Autodesk Inventor part; units mm, degrees
ref_plane "Work Plane2" through (-142.9124, -40, 12) normal (0, 0, 1) x (1, 0, 0)
ref_plane "YZ Plane" through (0, 0, 0) normal (1, 0, 0) x (0, 1, 0)
ref_plane "XZ Plane" through (0, 0, 0) normal (0, 1, 0) x (-1, 0, 0)
ref_plane "Work Plane1" through (0, 0, 0) normal (0, 0, 1) x (1, 0, 0)
sketch "Sketch1" plane through (0, 0, 0) normal (0, 0, 1) x (1, 0, 0)
  circle A0 centre (13.9438, -25.4) radius 3.3782 construction
  line L0 (31.1796, -40) -> (-0.106, -40) construction
  line L1 (31.1796, -40) -> (31.1796, -8.95) construction
  line L2 (31.1796, -8.95) -> (23.5548, -8.95) construction
  line L3 (23.5548, -8.95) -> (23.5548, -10.525) construction
  line L4 (23.5548, -10.525) -> (12.648, -10.525) construction
  line L5 (12.648, -10.525) -> (12.648, -8.95) construction
  line L6 (12.648, -8.95) -> (-0.106, -8.95) construction
  line L7 (-0.106, -8.95) -> (-0.106, -40) construction
  circle A1 centre (13.9438, 25.4) radius 3.3782 construction
  line L8 (-0.106, 8.95) -> (12.648, 8.95) construction
  line L9 (12.648, 8.95) -> (12.648, 10.525) construction
  line L10 (12.648, 10.525) -> (23.5548, 10.525) construction
  line L11 (23.5548, 10.525) -> (23.5548, 8.95) construction
  line L12 (23.5548, 8.95) -> (31.1796, 8.95) construction
  line L13 (31.1796, 8.95) -> (31.1796, 45) construction
  line L14 (-0.106, 45) -> (31.1796, 45) construction
  line L15 (-0.106, 45) -> (-0.106, 8.95) construction
  line L16 (31.1796, -18.5) -> (-0.106, -18.5)
  line L17 (-0.106, -18.5) -> (-0.106, 18.5)
  line L18 (-0.106, 18.5) -> (31.1796, 18.5)
  line L19 (31.1796, 18.5) -> (31.1796, -18.5)
  line L20 (65.998, 0) -> (-177.7308, 0) construction
  circle A2 centre (13.9438, 25.4) radius 5.5 construction
  circle A3 centre (23.1796, -13.5) radius 2
  circle A4 centre (7.894, -13.5) radius 2
  circle A5 centre (7.894, 13.5) radius 2
  circle A6 centre (23.1796, 13.5) radius 2
  point P0 (0, 0)
  point P1 (13.9438, 22.0218)
  dimension "d2" = 37
  dimension "d3" = 11
ref_plane "Work Plane2" through (-142.9124, -40, 12) normal (0, 0, 1) x (1, 0, 0)
extrude "Extrusion1" add sketch "Sketch1" along normal up to surface (12 mm away) contours L16 L17 L18 L19 | A3 | A4 | A5 | A6
sketch "Sketch2" plane through (0, 0, 0) normal (0, 1, 0) x (-1, 0, 0)
  line L0 (1.106, -8.95) -> (1.106, 0)
  line L1 (1.106, 0) -> (-32.1796, 0)
  line L2 (-32.1796, 0) -> (-32.1796, -8.95)
  line L3 (-38.8367, 0) -> (7.7631, 0) construction
  line L4 (-31.1796, -8.95) -> (-31.1796, 0) construction
  line L5 (0.106, 7.5245) -> (0.106, -7.5245) construction
  line L6 (-31.1796, -8.95) -> (-23.5548, -8.95)
  line L7 (-23.5548, -10.525) -> (-12.648, -10.525)
  line L8 (-12.648, -8.95) -> (0.106, -8.95)
  line L9 (-31.1796, -8.95) -> (-32.1796, -8.95)
  line L10 (0.106, -8.95) -> (1.106, -8.95)
  line L11 (-23.5548, -8.95) -> (-23.5548, -10.525)
  line L12 (-12.648, -8.95) -> (-12.648, -10.525)
  point P0 (0, 0)
  point P1 (1.106, 0)
  point P2 (-32.1796, 0)
  dimension "d7" = 1
  dimension "d8" = 1
revolve "Revolution1" cut sketch "Sketch2" angle 360 about axis through (0, 0, 0) along (-1, 0, 0)
sketch "Sketch3" plane through (0, 0, 0) normal (0, 0, -1) x (-1, 0, 0)
  line L0 (0.106, 18.5) -> (-31.1796, 18.5)
  line L1 (-31.1796, 18.5) -> (-31.1796, -18.5)
  line L2 (-31.1796, -18.5) -> (0.106, -18.5)
  line L3 (0.106, -18.5) -> (0.106, 18.5)
  point P0 (0, 0)
extrude "Extrusion2" cut sketch "Sketch3" against normal blind 0.2
sketch "Sketch4" plane through (-0.106, 18.5, 12) normal (0, 0, 1) x (1, 0, 0)
  line L0 (31.2856, 0) -> (31.2856, -37) construction
  line L1 (0, 0) -> (31.2856, 0) construction
  line L2 (0, -37) -> (0, 0) construction
  line L3 (31.2856, -37) -> (0, -37) construction
  line L4 (31.2856, -5) -> (0, -5) construction
  line L5 (-6.2571, -18.5) -> (37.5427, -18.5) construction
  line L6 (31.2856, 0) -> (31.2856, -37) construction
  line L7 (0, -37) -> (0, 0) construction
  point P0 (0.106, -18.5)
  point P1 (23.2856, -5)
  point P2 (8, -5)
  point P3 (23.2856, -32)
  point P4 (8, -32)
  dimension "d12" = 8
  dimension "d13" = 8
  dimension "d14" = 5
hole "Thru Hole Holddown Screws M3" at (23.1796, 13.5, 12) at (7.894, 13.5, 12) at (23.1796, -13.5, 12) at (7.894, -13.5, 12) direction (0, 0, -1) diameter 3.5 end through all
properties part number "Cuvette Holder Transmit Holddown"
Model file for the job. Use its own axes, mm. A direction names the side the tool comes from. Coordinates: 2 decimals unless noted, no trailing zeros. Order: outer loops, then holes, each group sorted by start corner. A loop starts at its lowest first (then second) coordinate and runs counter-clockwise, first axis right, second up. Notation, with made-up numbers: (36, -29) -> (46, -29) arc R16 cw to (46, -20) -> close; hole circle Ø10 at (12.25, 61). An arc over 180 degrees is marked (long way). Return JSON: item names as keys, results as strings.
Item 1: Slice it at D-D (y = -13.5). Write the cut outline in (x, z).
Model answer:
{"outline": "(-0.11, 0.2) -> (6.14, 0.2) -> (6.14, 12) -> (-0.11, 12) -> close; (9.64, 0.2) -> (21.43, 0.2) -> (21.43, 12) -> (9.64, 12) -> close; (24.93, 0.2) -> (31.18, 0.2) -> (31.18, 12) -> (24.93, 12) -> close"}
Item 2: Wall check: line 1 along X through (y, z) = (13.5, 9); line 2 along Y through (x, z) = (22.5, 6.25); line 3 along Y through (x, z) = (7, 6.75). Give the ranges that are in metal, low to high. Write a range as from..to.
Model answer:
{"line 1": "x = -0.11..6.14, 9.64..21.43, 24.93..31.18", "line 2": "y = -18.5..-15.11, -11.89..-8.47, 8.47..11.89, 15.11..18.5", "line 3": "y = -18.5..-15, -12..-5.88, 5.88..12, 15..18.5"}
Item 3: Mould opens along X. For faces 3 (the face through (-0.106, 0, 10)), 4 (the face through (8.6, 11.9, 6)), 5 (the face through (16, -18.5, 6)) say: pulls with the +X half, pulls with the -X half, needs draft (parallel to the pull), parting line crosses it, or undercut.
Model answer:
{"face 3": "pulls with the -X half", "face 4": "undercut", "face 5": "needs draft"}
Item 4: Slice it at C-C (y = 0). Write the cut outline in (x, z) (3 decimals).
Model answer:
{"outline": "(-0.106, 8.95) -> (12.648, 8.95) -> (12.648, 10.525) -> (23.555, 10.525) -> (23.555, 8.95) -> (31.18, 8.95) -> (31.18, 12) -> (-0.106, 12) -> close"}
Item 5: Slice it at A-A (z = 8.25). Write the cut outline in (x, y), then the cut area to 3 significant figures.
Model answer:
{"outline": "(-0.11, -18.5) -> (31.18, -18.5) -> (31.18, -3.47) -> (23.55, -3.47) -> (23.55, -6.54) -> (12.65, -6.54) -> (12.65, -3.47) -> (-0.11, -3.47) -> close; (-0.11, 3.47) -> (12.65, 3.47) -> (12.65, 6.54) -> (23.55, 6.54) -> (23.55, 3.47) -> (31.18, 3.47) -> (31.18, 18.5) -> (-0.11, 18.5) -> close; hole circle Ø3.5 at (7.89, -13.5); hole circle Ø3.5 at (7.89, 13.5); hole circle Ø3.5 at (23.18, -13.5); hole circle Ø3.5 at (23.18, 13.5)", "area": "835 mm²"}
Item 6: 3-axis set-ups, long thin cutter, end or side, ignore diameter. For faces 1 (the face through (23.555, 2, 9)), 2 (the face through (6.182, -0.194, 8.948)): which of +Z, -Z, +X, -X, +Y, -Y reach the whole face in a straight line?
Model answer:
{"face 1": "-Z", "face 2": "-Z, +X, -X"}
